Autodesk Inventor part; units mm, degrees
ref_plane "YZ Plane" through (0, 0, 0) normal (1, 0, 0) x (0, 1, 0)
ref_plane "XZ Plane" through (0, 0, 0) normal (0, 1, 0) x (-1, 0, 0)
ref_plane "XY Plane" through (0, 0, 0) normal (0, 0, 1) x (1, 0, 0)
sketch "Sketch1" plane through (0, 0, 0) normal (1, 0, 0) x (0, 1, 0)
  line L0 (0, 0) -> (7, 0)
  line L1 (0, 0) -> (0, -15) construction
  line L2 (0, -4) -> (5, -4)
  line L3 (5, -4) -> (5, -5)
  line L4 (5, -5) -> (0, -5)
  line L5 (0, -5) -> (0, -4)
  circle A0 centre (2.5, -6.4) radius 2.2
  line L6 (2.5, 0) -> (2.5, -6.4) construction
  point P0 (0.8029, -5)
  point P1 (4.1971, -5)
  dimension "d2" = 7
  dimension "d3" = 15
  dimension "d4" = 5
  dimension "d5" = 8
  dimension "d6" = 4.4
  dimension "d7" = 2.5
  dimension "d8" = 1.4
  dimension "d9" = 1
revolve "Revolution1" add sketch "Sketch1" angle 360 about axis through (0, 0, 0) along (0, 1, 0) contours L2 L3 L4 A0 L5
chamfer "Chamfer1" distance 0.25 angle 45 2 edges at (0, 5, 5) (0, 0, 5)
properties part number "Inner_Ring"
Geometry: final body of the model. Coordinates: model frame, mm. Give positions to 0.01 mm unless a question says otherwise; leave off trailing zeros. Write each loop counter-clockwise with the first axis right and the second up, starting at its lowest first coordinate (ties: lowest second). Pieces come first, ordered by that corner, then holes.
1. Section query B-B, the plane z = 0. Return loops of the section in (x, y).
2. Section query A-A, the plane x = 0. Return loops of the section in (y, z).
3. Line query: probe 1 along X at (y, z) = (0.45, 1.5); probe 2 along X at (y, z) = (3.15, 0); probe 3 along Z at (x, y) = (0, 3.7). Output: solid intervals per line, ascending.
4. Section query D-D, the plane y = 1.55. Return loops of the section in (x, z).
5. Section query C-C, the plane y = 4.6. Return loops of the section in (x, z).
6. Pin query (flat end, axial travel): P1, Ø1.5, axis at y = 2, z = -2.5, coming from the -X side; P2, Ø1.5, axis at y = 2, z = -1, coming from the -X side; P3, Ø1, axis at y = 1, z = 2, coming from the +X side. Return the tip coordinate at first contact, or that it passes through.
7. Draft query along Z for faces 1 (the cylindrical face through (-4.88, 0.52, 1.08)), 2 (the cylindrical face through (3.905, 2.535, 0.867)), 3 (the flat face through (2, 0, 4)). Return one class per face: released by +Z, released by -Z, zero draft, split by the parting line, or undercut.
Computed:
1. outline: (-5, 0.25) - (-4.75, 0) - (-4, 0) - (-4, 5) - (-4.75, 5) - (-5, 4.75) - (-5, 4.2) arc R2.2 cw to (-5, 0.8) - close; (4, 0) - (4.75, 0) - (5, 0.25) - (5, 0.8) arc R2.2 cw to (5, 4.2) - (5, 4.75) - (4.75, 5) - (4, 5) - close
2. outline: (0, -4.75) - (0.25, -5) - (0.8, -5) arc R2.2 cw to (4.2, -5) - (4.75, -5) - (5, -4.75) - (5, -4) - (0, -4) - close; (0, 4) - (5, 4) - (5, 4.75) - (4.75, 5) - (4.2, 5) arc R2.2 cw to (0.8, 5) - (0.25, 5) - (0, 4.75) - close
3. probe 1: x = -4.77 to -3.71, 3.71 to 4.77
3. probe 2: x = -4.3 to -4, 4 to 4.3
3. probe 3: z = -4.56 to -4, 4 to 4.56
4. outline: circle Ø8.83 at (0, 0); hole circle Ø8 at (0, 0)
5. outline: circle Ø10 at (0, 0); hole circle Ø8 at (0, 0)
6. P1: stops at x = -4
6. P2: stops at x = -4.5
6. P3: stops at x = 4.76
7. face 1: split by the parting line
7. face 2: undercut
7. face 3: zero draft
